Design review of the part shown in the three views and the two pictorial views. Dimensions are in mm from the part's minimum x, y and z. A direction names the side the tool comes from. Round coordinates to 2 decimals unless told otherwise and drop trailing zeros. Order: outer loops, then holes, each group sorted by start corner. A loop starts at its lowest first (then second) coordinate and runs counter-clockwise, first axis right, second up.
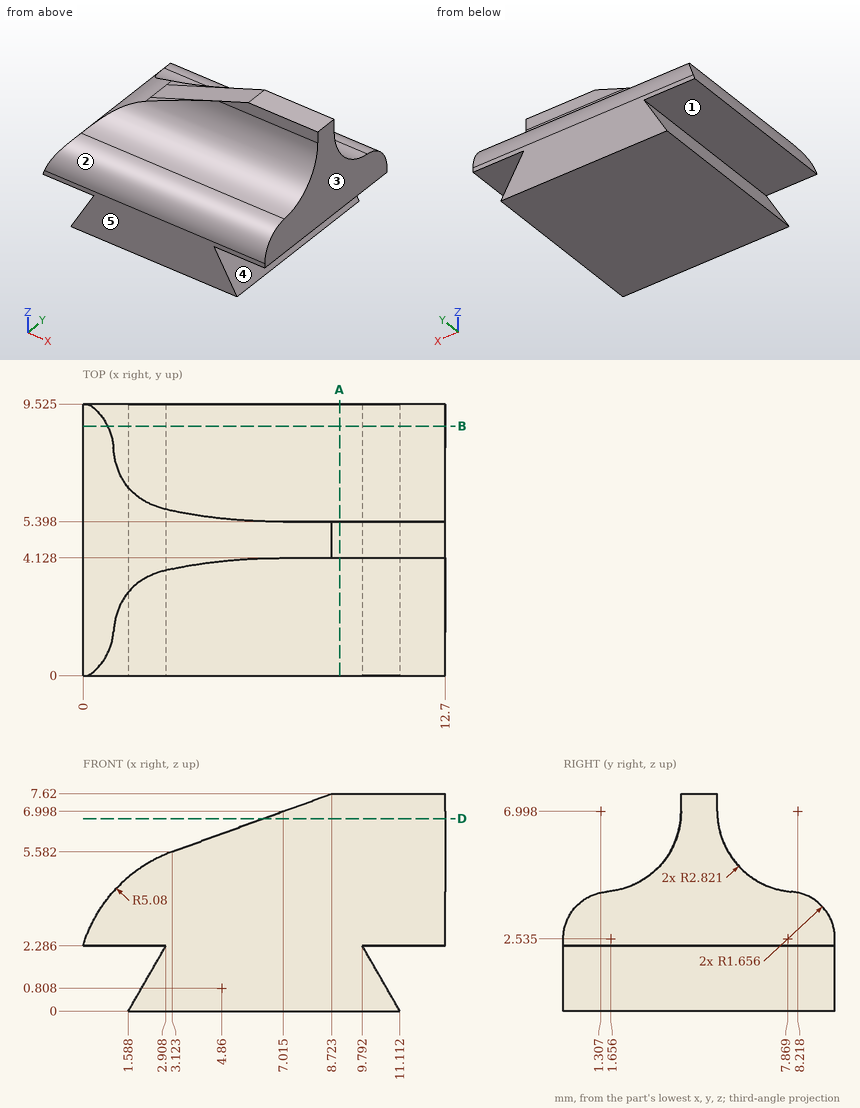
1) Take a section at D-D on z = 6.75. Give the boundary of the cut face in (x, y).
Results:
outline: (6.33, 4.12) - (12.7, 4.12) - (12.7, 5.41) - (6.33, 5.41) - close
2) Clearance check with flat-ended pins moving along their axes: P1, Ø1, axis at x = 5, z = 5, coming from the -Y side (1 decimal); P2, Ø4, axis at x = 10.5, z = 6.5, coming from the +Y side (1 decimal). State where each tip first meets the part, or that it passes through.
Results:
P1: stops at y = 2.6
P2: stops at y = 6.9
3) Take a section at B-B on y = 8.75. Give the boundary of the cut face in (x, z) (1 decimal).
Results:
outline: (0, 2.3) - (2.9, 2.3) - (1.6, 0) - (11.1, 0) - (9.8, 2.3) - (12.7, 2.3) - (12.7, 3.9) - (0.9, 3.9) arc R5.1 ccw to start
4) For the marked faces 4 and 5, list the 3-axis set-ups (+Z, -Z, +X, -X, +Y, -Y) from which the entire face can be reached by the end or side of a thin tool; tool diameter is ignored.
Results:
face 4: +X, +Y, -Y
face 5: +Z, -Z, +X, -X, -Y
5) To check wall thickness, follow line 1 along Z through (x, y) = (7.25, 8) (1 decimal); line 2 along Z through (x, y) = (10.5, 6.75) (1 decimal); line 3 along Z through (x, y) = (9.5, 9) (1 decimal). State the ranges of each line that lie inside material, in increasing order.
Results:
line 1: z = 0 to 4.2
line 2: z = 0 to 1.1, 2.3 to 4.6
line 3: z = 0 to 3.7
6) The part is to be moulded in two halves that separate along Z. For the marked faces 1, 2 and 3, say which applies: released by +Z, released by -Z, zero draft, split by the parting line, or undercut.
Results:
face 1: undercut
face 2: released by +Z
face 3: zero draft
7) Take a section at A-A on x = 9. Give the boundary of the cut face in (y, z) (1 decimal).
Results:
outline: (0, 0) - (9.5, 0) - (9.5, 2.5) arc R1.7 ccw to (8, 4.2) arc R2.8 cw to (5.4, 7) - (5.4, 7.6) - (4.1, 7.6) - (4.1, 7) arc R2.8 cw to (1.5, 4.2) arc R1.7 ccw to (0, 2.5) - close
